Check sheet for the modelled part. Datum: model origin and axes. Units: mm. Face numbers are marked on the shaded views. A direction names the side the tool comes from. Round coordinates to 2 decimals unless told otherwise and drop trailing zeros. Order: outer loops, then holes, each group sorted by start corner. A loop starts at its lowest first (then second) coordinate and runs counter-clockwise, first axis right, second up. Notation, with made-up numbers: (-34, 43.25) -> (-9, 43.25) arc R21 cw to (-9, 78.25) -> close; hole circle Ø8 at (16, 0.25). An arc over 180 degrees is marked (long way). Use CSV: the item, a comma, the result in double quotes.
```python
from build123d import *

# Parameters (mm, degrees)
SKETCH1_W           = 57
SKETCH1_H           = 57
SKETCH1_R           = 2.65
BOSS_EXTRUDE1_DEPTH = 113
SKETCH2_R           = 19.075
BOSS_EXTRUDE2_DEPTH = 1.6
SKETCH3_R           = 5
BOSS_EXTRUDE3_DEPTH = 22.4


with BuildPart() as part:
    # Sketch1 → Boss-Extrude1 (new body)
    with BuildSketch(Plane.XY):
        Rectangle(SKETCH1_W, SKETCH1_H)
        with Locations((-23.5, 23.5)):
            Circle(SKETCH1_R, mode=Mode.SUBTRACT)
        with Locations((23.5, 23.5)):
            Circle(SKETCH1_R, mode=Mode.SUBTRACT)
        with Locations((23.5, -23.5)):
            Circle(SKETCH1_R, mode=Mode.SUBTRACT)
        with Locations((-23.5, -23.5)):
            Circle(SKETCH1_R, mode=Mode.SUBTRACT)
    extrude(amount=BOSS_EXTRUDE1_DEPTH)

    # Sketch2 → Boss-Extrude2 (add)
    with BuildSketch(Plane.XY):
        Circle(SKETCH2_R)
    extrude(amount=-BOSS_EXTRUDE2_DEPTH)

    # Sketch3 → Boss-Extrude3 (add)
    with BuildSketch(Plane.XY):
        Circle(SKETCH3_R)
    extrude(amount=-BOSS_EXTRUDE3_DEPTH)


solid = part.part
```
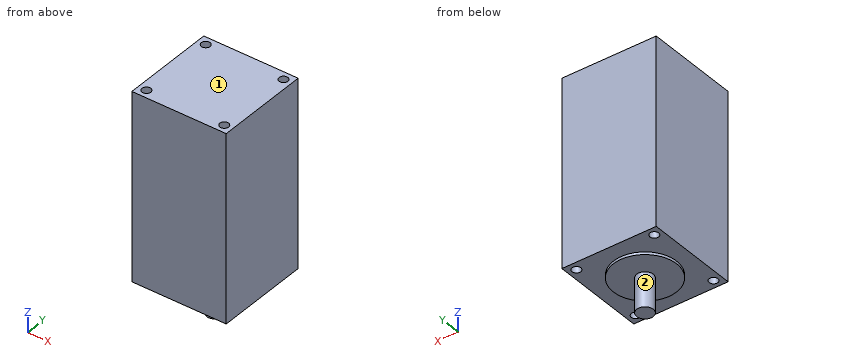
Q1. Sectioned sample at D-D, the plane x = 0. Enter the section's corners in (y, z) (3 decimals).
Result sheet:
outline,"(-28.5, 0) -> (-19.075, 0) -> (-19.075, -1.6) -> (-5, -1.6) -> (-5, -22.4) -> (5, -22.4) -> (5, -1.6) -> (19.075, -1.6) -> (19.075, 0) -> (28.5, 0) -> (28.5, 113) -> (-28.5, 113) -> close"
Q2. Access from +Z, -Z, +X, -X, +Y, -Y to the whole of each face (thin tool, end or side, straight path). Record for the marked faces 1 and 2.
Result sheet:
face 1,"+Z, +X, -X, +Y, -Y"
face 2,"-Z"
Q3. Scan lines: L1, parallel to Y at x = -23.5, z = 64; L2, parallel to X at y = -25, z = 44; L3, parallel to X at y = 23, z = 49. Record each from-to range of solid material in increasing order.
Result sheet:
L1,"y = -28.5 to -26.15, -20.85 to 20.85, 26.15 to 28.5"
L2,"x = -28.5 to -25.68, -21.32 to 21.32, 25.68 to 28.5"
L3,"x = -28.5 to -26.1, -20.9 to 20.9, 26.1 to 28.5"
Q4. Go/stop test with flat-tipped pins: pin 1 (1.5 mm diameter, centred on x = 19, y = -5, fed in from -Z); pin 2 (7 mm diameter, centred on x = -23.5, y = -23.5, fed in from -Z). Record where each tip stops, or that it passes through.
Result sheet:
pin 1,"stops at z = -1.6"
pin 2,"stops at z = 0"
Q5. Sectioned sample at A-A, the plane y = 23.5. Enter the section's corners in (x, z), then the cut area to 3 significant figures.
Result sheet:
outline,"(-28.5, 0) -> (-26.15, 0) -> (-26.15, 113) -> (-28.5, 113) -> close; (-20.85, 0) -> (20.85, 0) -> (20.85, 113) -> (-20.85, 113) -> close; (26.15, 0) -> (28.5, 0) -> (28.5, 113) -> (26.15, 113) -> close"
area,"5,240 mm^2"
Q6. Sectioned sample at C-C, the plane z = 87. Enter the section's corners in (x, y), then the cut area to 3 significant figures.
Result sheet:
outline,"(-28.5, -28.5) -> (28.5, -28.5) -> (28.5, 28.5) -> (-28.5, 28.5) -> close; hole circle Ø5.3 at (-23.5, -23.5); hole circle Ø5.3 at (-23.5, 23.5); hole circle Ø5.3 at (23.5, -23.5); hole circle Ø5.3 at (23.5, 23.5)"
area,"3,160 mm^2"
